The model under review builds one solid part; all positions refer to its coordinate system, in mm. Coordinates: 2 decimals unless noted, no trailing zeros.
```python
from build123d import *

# Parameters (mm, degrees)
SKETCH1_R           = 2.1
BOSS_EXTRUDE1_DEPTH = 332.5
SKETCH2_W           = 11
SKETCH2_H           = 1.8
CUT_EXTRUDE1_DEPTH  = 272.5


with BuildPart() as part:
    # Sketch1 → Boss-Extrude1 (new, symmetric)
    with BuildSketch(Plane.XY):
        with BuildLine():
            Line((4.58, -20), (9.5, -20))
            ThreePointArc((9.5, -20), (9.853553391, -19.853553391), (10, -19.5))
            Line((10, -19.5), (10, -14.58))
            Line((10, -14.58), (8.545, -13.125))
            Line((8.545, -13.125), (8.2, -13.125))
            Line((8.2, -13.125), (8.2, -15.5))
            Line((8.2, -15.5), (6.560660172, -15.5))
            Line((6.560660172, -15.5), (3.9, -12.839339828))
            Line((3.9, -12.839339828), (3.9, -10.21))
            Line((3.9, -10.21), (3.69, -10))
            Line((3.69, -10), (3.9, -9.79))
            Line((3.9, -9.79), (3.9, -7.160660172))
            Line((3.9, -7.160660172), (6.560660172, -4.5))
            Line((6.560660172, -4.5), (8.2, -4.5))
            Line((8.2, -4.5), (8.2, -6.875))
            Line((8.2, -6.875), (8.545, -6.875))
            Line((8.545, -6.875), (10, -5.42))
            Line((10, -5.42), (10, 5.42))
            Line((10, 5.42), (8.545, 6.875))
            Line((8.545, 6.875), (8.2, 6.875))
            Line((8.2, 6.875), (8.2, 4.5))
            Line((8.2, 4.5), (6.560660172, 4.5))
            Line((6.560660172, 4.5), (3.9, 7.160660172))
            Line((3.9, 7.160660172), (3.9, 9.79))
            Line((3.9, 9.79), (3.69, 10))
            Line((3.69, 10), (3.9, 10.21))
            Line((3.9, 10.21), (3.9, 12.839339828))
            Line((3.9, 12.839339828), (6.560660172, 15.5))
            Line((6.560660172, 15.5), (8.2, 15.5))
            Line((8.2, 15.5), (8.2, 13.125))
            Line((8.2, 13.125), (8.545, 13.125))
            Line((8.545, 13.125), (10, 14.58))
            Line((10, 14.58), (10, 19.5))
            ThreePointArc((10, 19.5), (9.853553391, 19.853553391), (9.5, 20))
            Line((9.5, 20), (4.58, 20))
            Line((4.58, 20), (3.125, 18.545))
            Line((3.125, 18.545), (3.125, 18.2))
            Line((3.125, 18.2), (5.5, 18.2))
            Line((5.5, 18.2), (5.5, 16.560660172))
            Line((5.5, 16.560660172), (2.839339828, 13.9))
            Line((2.839339828, 13.9), (0.21, 13.9))
            Line((0.21, 13.9), (0, 13.69))
            Line((0, 13.69), (-0.21, 13.9))
            Line((-0.21, 13.9), (-2.839339828, 13.9))
            Line((-2.839339828, 13.9), (-5.5, 16.560660172))
            Line((-5.5, 16.560660172), (-5.5, 18.2))
            Line((-5.5, 18.2), (-3.125, 18.2))
            Line((-3.125, 18.2), (-3.125, 18.545))
            Line((-3.125, 18.545), (-4.58, 20))
            Line((-4.58, 20), (-9.5, 20))
            ThreePointArc((-9.5, 20), (-9.853553391, 19.853553391), (-10, 19.5))
            Line((-10, 19.5), (-10, 14.58))
            Line((-10, 14.58), (-8.545, 13.125))
            Line((-8.545, 13.125), (-8.2, 13.125))
            Line((-8.2, 13.125), (-8.2, 15.5))
            Line((-8.2, 15.5), (-6.560660172, 15.5))
            Line((-6.560660172, 15.5), (-3.9, 12.839339828))
            Line((-3.9, 12.839339828), (-3.9, 10.21))
            Line((-3.9, 10.21), (-3.69, 10))
            Line((-3.69, 10), (-3.9, 9.79))
            Line((-3.9, 9.79), (-3.9, 7.160660172))
            Line((-3.9, 7.160660172), (-6.560660172, 4.5))
            Line((-6.560660172, 4.5), (-8.2, 4.5))
            Line((-8.2, 4.5), (-8.2, 6.875))
            Line((-8.2, 6.875), (-8.545, 6.875))
            Line((-8.545, 6.875), (-10, 5.42))
            Line((-10, 5.42), (-10, -5.42))
            Line((-10, -5.42), (-8.545, -6.875))
            Line((-8.545, -6.875), (-8.2, -6.875))
            Line((-8.2, -6.875), (-8.2, -4.5))
            Line((-8.2, -4.5), (-6.560660172, -4.5))
            Line((-6.560660172, -4.5), (-3.9, -7.160660172))
            Line((-3.9, -7.160660172), (-3.9, -9.79))
            Line((-3.9, -9.79), (-3.69, -10))
            Line((-3.69, -10), (-3.9, -10.21))
            Line((-3.9, -10.21), (-3.9, -12.839339828))
            Line((-3.9, -12.839339828), (-6.560660172, -15.5))
            Line((-6.560660172, -15.5), (-8.2, -15.5))
            Line((-8.2, -15.5), (-8.2, -13.125))
            Line((-8.2, -13.125), (-8.545, -13.125))
            Line((-8.545, -13.125), (-10, -14.58))
            Line((-10, -14.58), (-10, -19.5))
            ThreePointArc((-10, -19.5), (-9.853553391, -19.853553391), (-9.5, -20))
            Line((-9.5, -20), (-4.58, -20))
            Line((-4.58, -20), (-3.125, -18.545))
            Line((-3.125, -18.545), (-3.125, -18.2))
            Line((-3.125, -18.2), (-5.5, -18.2))
            Line((-5.5, -18.2), (-5.5, -16.560660172))
            Line((-5.5, -16.560660172), (-2.839339828, -13.9))
            Line((-2.839339828, -13.9), (-0.21, -13.9))
            Line((-0.21, -13.9), (0, -13.69))
            Line((0, -13.69), (0.21, -13.9))
            Line((0.21, -13.9), (2.839339828, -13.9))
            Line((2.839339828, -13.9), (5.5, -16.560660172))
            Line((5.5, -16.560660172), (5.5, -18.2))
            Line((5.5, -18.2), (3.125, -18.2))
            Line((3.125, -18.2), (3.125, -18.545))
            Line((3.125, -18.545), (4.58, -20))
        make_face()
        with Locations((0, -10)):
            Circle(SKETCH1_R, mode=Mode.SUBTRACT)
        Polygon((-6.239339828, -2.7), (-8.2, -2.7), (-8.2, 2.7), (-6.239339828, 2.7), (-2.839339828, 6.1), (2.839339828, 6.1), (6.239339828, 2.7), (8.2, 2.7), (8.2, -2.7), (6.239339828, -2.7), (2.839339828, -6.1), (-2.839339828, -6.1), align=None, mode=Mode.SUBTRACT)
        with Locations((0, 10)):
            Circle(SKETCH1_R, mode=Mode.SUBTRACT)
    extrude(amount=BOSS_EXTRUDE1_DEPTH, both=True)

    # Sketch2 → Cut-Extrude1 (cut, symmetric)
    with BuildSketch(Plane.XY):
        with Locations((0, -19.1)):
            Rectangle(SKETCH2_W, SKETCH2_H)
    cut_extrude1 = extrude(amount=CUT_EXTRUDE1_DEPTH, both=True, mode=Mode.SUBTRACT)

    # Mirror1: Cut-Extrude1 across plane
    add(cut_extrude1.mirror(Plane.ZX), mode=Mode.SUBTRACT)


solid = part.part
```
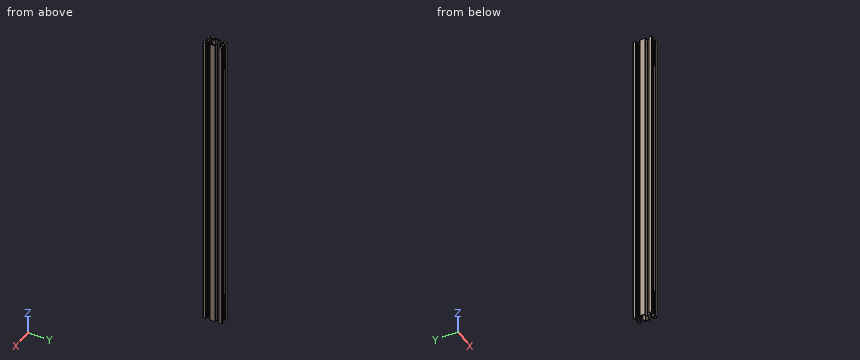
Item 1: Take a section at A-A, the plane z = -89. Count the separate pieces of the cut face and the enclosed holes in it, plus the area to 3 significant figures.
Solved:
separate pieces: 1
enclosed holes: 3
area: 287 mm2
Item 2: For pin 1 (6 mm diameter, centred on x = 5, z = -259, fed in from +Y); pin 2 (0.8 mm diameter, centred on y = -12, z = 60.5, fed in from -X); pin 3 (0.7 mm diameter, centred on y = -14, z = 70.5, fed in from +X); pin 4 (2 mm diameter, centred on x = -1.5, z = 9.5, fed in from -Y), all flat-tipped, find the tip position at first contact; note any pin that passes through.
Solved:
pin 1: stops at y = 20
pin 2: stops at x = -3.9
pin 3: stops at x = 9.77
pin 4: stops at y = -13.9
Item 3: To check wall thickness, follow line 1 along Y through (x, z) = (0, 21); line 2 along X through (y, z) = (-3.5, 152); line 3 along Y through (x, z) = (7.75, -100.5). State the ranges of each line that lie inside material, in increasing order.
Solved:
line 1: y = -13.69 to -12.1, -7.9 to -6.1, 6.1 to 7.9, 12.1 to 13.69
line 2: x = -10 to -5.44, 5.44 to 10
line 3: y = -20 to -15.5, -4.5 to -2.7, 2.7 to 4.5, 15.5 to 20
